Read the model definition and answer for the solid it produces. Units are mm, in the model's axes. Give positions to 0.01 mm unless a question says otherwise; leave off trailing zeros. Order: outer loops, then holes, each group sorted by start corner. A loop starts at its lowest first (then second) coordinate and runs counter-clockwise, first axis right, second up. Notation, with made-up numbers: (54.25, 49) - (76.25, 49) arc R8 cw to (76.25, 64) - close; hole circle Ø8 at (86.25, -2.75). An arc over 180 degrees is marked (long way). One line per item, written item: value. Start each with the question number.
```python
from build123d import *

# Parameters (mm, degrees)
F0_W        = 50.8
F0_H        = 3.0988
F1_DEPTH    = 7.62
F3_T1_DEPTH = 69.5151640121
F4_DEPTH    = 25.4


# Not quite as in the source:
# - a fillet or chamfer that OpenCascade refuses, or shapes differently, is made with other operations: its cross-section is extruded or revolved along the edge and cut away or added


with BuildPart() as f1:
    # F0 (on Top) → F1 (new body)
    with BuildSketch(Plane.XY):
        with Locations((0, 1.5494)):
            Rectangle(F0_W, F0_H)
    extrude(amount=F1_DEPTH)

    # F3: fillet of radius 3.81 on 1 edges, made by hand

    # F3_s2 → F3_t1 (cut)
    with BuildSketch(Plane.YZ.offset(-34.7575820061)):
        with BuildLine():
            ThreePointArc((0, 3.8769671976), (0.8752281179, 6.3066202592), (3.0988, 7.62))
            Line((3.0988, 7.62), (0, 7.62))
            Line((0, 7.62), (0, 3.8769671976))
        make_face()
    extrude(amount=F3_T1_DEPTH, mode=Mode.SUBTRACT)

    # F2 (on face) → F4 (cut)
    with BuildSketch(Plane.XZ):
        Polygon((-22.225, 6.3092954744), (-21.4682643893, 7.62), (-22.9817356107, 7.62), align=None)
        Polygon((-12.5782643893, 7.62), (-14.0917356107, 7.62), (-13.335, 6.3092954744), align=None)
        Polygon((14.2383825791, 7.62), (12.4316174209, 7.62), (13.335, 6.0552954744), align=None)
        Polygon((22.225, 5.9282954744), (23.2017060633, 7.62), (21.2482939367, 7.62), align=None)
        Polygon((-3.6882643893, 7.62), (-5.2017356107, 7.62), (-4.445, 6.3092954744), align=None)
        Polygon((5.2750590949, 7.62), (3.6149409051, 7.62), (4.445, 6.1822954744), align=None)
    extrude(amount=-F4_DEPTH, mode=Mode.SUBTRACT)


solid = f1.part
```
1) Section D-D on z = 4.5 is taken. Write down the section's boundary in (x, y).
2) This flat-tipped pin is pushed along its axis until it touches: pin 1 (1.5 mm diameter, centred on x = -20, y = 0.5, fed in from +Z). Where does it stop, or does it pass through?
3) Find the intervals of material crossed by probe 1 along Y at (x, z) = (-12, 4); probe 2 along Z at (x, y) = (-2, 0.95); probe 3 along Y at (x, z) = (6, 5.25), in increasing order. Write a range as from..to.
4) Section B-B on y = 1.9 is taken. Write down the section's boundary in (x, z) (3 decimals).
5) Section C-C on x = -18 is taken. Write down the section's boundary in (y, z), plus the area to 3 significant figures.
6) The mould has two halves that part along X. Classify faces 1 (the flat face through (-13.635, 2.219, 6.828)), 2 (the flat face through (0, 0, 2)), 3 (the flat face through (25.4, 2, 4)): +X half, -X half, draft (parallel to the pull), parting line (faces both ways), or undercut.
7) Section A-A on z = 6.75 is taken. Write down the section's boundary in (x, y), plus the area to 3 significant figures.
Solved:
1. outline: (-25.4, 0.05) - (25.4, 0.05) - (25.4, 3.1) - (-25.4, 3.1) - close
2. pin 1: stops at z = 6.7
3. probe 1: y = 0..3.1
3. probe 2: z = 0..6.39
3. probe 3: y = 0.26..3.1
4. outline: (-25.4, 0) - (25.4, 0) - (25.4, 7.174) - (22.944, 7.174) - (22.225, 5.928) - (21.506, 7.174) - (13.981, 7.174) - (13.335, 6.055) - (12.689, 7.174) - (5.017, 7.174) - (4.445, 6.182) - (3.873, 7.174) - (-3.946, 7.174) - (-4.445, 6.309) - (-4.944, 7.174) - (-12.836, 7.174) - (-13.335, 6.309) - (-13.834, 7.174) - (-21.726, 7.174) - (-22.225, 6.309) - (-22.724, 7.174) - (-25.4, 7.174) - close
5. outline: (0, 0) - (3.1, 0) - (3.1, 7.62) arc R3.81 ccw to (0, 3.88) - close
5. area: 20.7 mm2
6. face 1: undercut
6. face 2: draft
6. face 3: +X half
7. outline: (-25.4, 1.31) - (-22.48, 1.31) - (-22.48, 3.1) - (-25.4, 3.1) - close; (-21.97, 1.31) - (-13.59, 1.31) - (-13.59, 3.1) - (-21.97, 3.1) - close; (-13.08, 1.31) - (-4.7, 1.31) - (-4.7, 3.1) - (-13.08, 3.1) - close; (-4.19, 1.31) - (4.12, 1.31) - (4.12, 3.1) - (-4.19, 3.1) - close; (4.77, 1.31) - (12.93, 1.31) - (12.93, 3.1) - (4.77, 3.1) - close; (13.74, 1.31) - (21.75, 1.31) - (21.75, 3.1) - (13.74, 3.1) - close; (22.7, 1.31) - (25.4, 1.31) - (25.4, 3.1) - (22.7, 3.1) - close
7. area: 83.9 mm2
